from build123d import *

# Parameters (mm, degrees)
F0_R      = 14
F0_R_2    = 3.15
F1_DEPTH  = 4
F2_R      = 9
F3_DEPTH  = 6
F4_R      = 8
F5_DEPTH  = 22
F6_R      = 6.5
F7_DEPTH  = 25
F10_DEPTH = 2
F11_DEPTH = 25
F9_R      = 5.35
F9_R_2    = 3.15
F12_DEPTH = 10


# Not quite as in the source:
# - a fillet or chamfer that OpenCascade refuses, or shapes differently, is made with other operations: its cross-section is extruded or revolved along the edge and cut away or added


with BuildPart() as f1:
    # F0 (on Top) → F1 (new body)
    with BuildSketch(Plane.XY):
        Circle(F0_R)
        Circle(F0_R_2, mode=Mode.SUBTRACT)
    extrude(amount=F1_DEPTH)

    # F2 (on Top) → F3 (join)
    with BuildSketch(Plane.XY):
        Circle(F2_R)
    extrude(amount=F3_DEPTH)

    # F4 (on Top) → F5 (join)
    with BuildSketch(Plane.XY):
        Circle(F4_R)
    extrude(amount=F5_DEPTH)

    # F6 (on Top) → F7 (cut)
    with BuildSketch(Plane.XY):
        Circle(F6_R)
    extrude(amount=F7_DEPTH, mode=Mode.SUBTRACT)

    # F0 (on Top) → F10 (join)
    with BuildSketch(Plane.XY):
        Circle(F0_R)
        Circle(F0_R_2, mode=Mode.SUBTRACT)
    extrude(amount=F10_DEPTH)

    # F8 (on Top) → F11 (cut)
    with BuildSketch(Plane.XY):
        with BuildLine():
            Line((3.9571776785, -10.1563155141), (2.7867408683, -9.2181909629))
            ThreePointArc((2.7867408683, -9.2181909629), (3.460013327, -11.5715284336), (5.4571776785, -10.1563155141))
            ThreePointArc((5.4571776785, -10.1563155141), (5.0953410965, -9.1792873497), (4.1843989666, -8.6736252274))
            Line((4.1843989666, -8.6736252274), (3.9571776785, -10.1563155141))
        make_face()
        with BuildLine():
            ThreePointArc((4.1843989666, -8.6736252274), (3.4126119429, -8.7586574158), (2.7867408683, -9.2181909629))
            Line((2.7867408683, -9.2181909629), (3.9571776785, -10.1563155141))
            Line((3.9571776785, -10.1563155141), (4.1843989666, -8.6736252274))
        make_face()
        with BuildLine():
            Line((-9.6037792731, 0.7130168091), (-10.7742160833, 1.6511413602))
            Line((-10.7742160833, 1.6511413602), (-9.376557985, 2.1957070958))
            ThreePointArc((-9.376557985, 2.1957070958), (-12.2569063699, 1.8783626483), (-9.6037792731, 0.7130168091))
        make_face()
        with BuildLine():
            Line((-9.376557985, 2.1957070958), (-10.7742160833, 1.6511413602))
            Line((-10.7742160833, 1.6511413602), (-9.6037792731, 0.7130168091))
            ThreePointArc((-9.6037792731, 0.7130168091), (-9.3590031637, 1.1539770087), (-9.2742160833, 1.6511413602))
            ThreePointArc((-9.2742160833, 1.6511413602), (-9.3000235674, 1.9281908617), (-9.376557985, 2.1957070958))
        make_face()
        with BuildLine():
            ThreePointArc((8.3170384048, 8.5051741539), (6.5399889033, 9.9793666697), (5.4193803065, 7.9606084183))
            Line((5.4193803065, 7.9606084183), (6.8170384048, 8.5051741539))
            Line((6.8170384048, 8.5051741539), (6.5898171167, 7.0224838672))
            ThreePointArc((6.5898171167, 7.0224838672), (7.7940665691, 7.3670107359), (8.3170384048, 8.5051741539))
        make_face()
        with BuildLine():
            Line((6.8170384048, 8.5051741539), (5.4193803065, 7.9606084183))
            ThreePointArc((5.4193803065, 7.9606084183), (5.8789138537, 7.3347373437), (6.5898171167, 7.0224838672))
            Line((6.5898171167, 7.0224838672), (6.8170384048, 8.5051741539))
        make_face()
    extrude(amount=F11_DEPTH, mode=Mode.SUBTRACT)

    # F9 (on Top) → F12 (join)
    with BuildSketch(Plane.XY):
        Circle(F9_R)
        Circle(F9_R_2, mode=Mode.SUBTRACT)
    extrude(amount=-F12_DEPTH)

    # F13: fillet of radius 5 on 1 edges, made by hand

    # F13_s1 → F13_t2 (revolve, cut)
    with BuildSketch(Plane.XZ):
        with BuildLine():
            ThreePointArc((8, 22), (6.8902277714, 20.3657774588), (6.5, 18.4292857857))
            Line((6.5, 18.4292857857), (6.5, 22))
            Line((6.5, 22), (8, 22))
        make_face()
    revolve(axis=Axis((0, 0, 22), (0, 0, -1)), mode=Mode.SUBTRACT)


solid = f1.part
Source: CAD feature listing. Evaluate the final solid. Frame: model axes, mm. A direction names the side the tool comes from. Coordinates: 2 decimals unless noted, no trailing zeros. Loops run counter-clockwise (first coordinate to the right, second up) from the corner with the lowest first, then second, coordinate; pieces in that order, holes last. Notation, with made-up numbers: (61.5, 74.5) - (70.5, 74.5) arc R17 ccw to (70.5, 84.5) - close; hole circle Ø11 at (-26.75, -9.5). An arc over 180 degrees is marked (long way). One line per question, with ' | ' between items.
1) Section C-C, the plane z = -7.5. Return loops of the section in (x, y).
Report:
outline: circle Ø10.7 at (0, 0); hole circle Ø6.3 at (0, 0)
2) Set-up query: faces 1 (the face through (12.932, -5.362, 1.972)), 2 (the face through (-1.16, -5.223, -4.93)), 3 (the face through (3, 2, 2)). Return all of +Z, -Z, +X, -X, +Y, -Y with unobstructed straight access to the full face (end or side cutting, diameter ignored); none if empty.
Report:
face 1: +Z, -Z | face 2: -Z | face 3: +Z
3) Section A-A, the plane z = 3.5. Return loops of the section in (x, y).
Report:
outline: circle Ø28 at (0, 0); hole circle Ø3 at (-10.77, 1.65); hole circle Ø13 at (0, 0); hole circle Ø3 at (3.96, -10.16); hole circle Ø3 at (6.82, 8.51)
4) Pull-direction query (X, two-part tool) for faces 4 (the face through (-5.158, -3.955, 10.1)), 5 (the face through (-3, -9, 4)), 6 (the face through (-1.73, -7.81, 13.89)); classes: released by +X, released by -X, zero draft, split by the parting line, or undercut.
Report:
face 4: undercut | face 5: zero draft | face 6: split by the parting line
5) Section B-B, the plane x = 0. Return loops of the section in (y, z).
Report:
outline: (-14, 0) - (-5.35, 0) - (-5.35, -10) - (-3.15, -10) - (-3.15, 2) - (-6.5, 2) - (-6.5, 18.43) arc R5 ccw to (-8, 22) - (-8, 6) - (-9, 6) - (-9, 4) - (-14, 4) - close; (3.15, -10) - (5.35, -10) - (5.35, 0) - (14, 0) - (14, 4) - (9, 4) - (9, 6) - (8, 6) - (8, 22) arc R5 ccw to (6.5, 18.43) - (6.5, 2) - (3.15, 2) - close
6) Section D-D, the plane z = 7. Return loops of the section in (x, y), then the cut area to 3 significant figures.
Report:
outline: circle Ø16 at (0, 0); hole circle Ø13 at (0, 0) | area: 68.3 mm²
7) First-contact query: P1, Ø15, axis at x = 0, y = 0, coming from the +Z side; P2, Ø2, axis at x = 11, z = 0.5, coming from the +Y side; P3, Ø6, axis at y = -4.5, z = -1, coming from the +X side. Flat tips, straight axial feed; report the tip coordinate or a pass-through.
Report:
P1: stops at z = 21.43 | P2: stops at y = 9.8 | P3: stops at x = 13.9
8) Line query: line 1 along X through (y, z) = (0, 10.75); line 2 along Z through (x, y) = (5.25, -7). Output: solid intervals per line, ascending.
Report:
line 1: x = -8 to -6.5, 6.5 to 8 | line 2: z = 0 to 6
